```python
from build123d import *

# Parameters (mm, degrees)
PAD002_DEPTH                  = 15.24
SKETCH006_W                   = 33.02
SKETCH006_H                   = 11.684
POCKET003_DEPTH               = 50.8
SKETCH007_R                   = 1.905
POCKET004_DEPTH               = 15.241
SKETCH008_R                   = 1.397
POCKET005_DEPTH               = 12.7
PAD003_DEPTH                  = 0.508
POCKET006_DEPTH               = 13.716
POCKET006_MIRRORED002_2_DEPTH = 13.716
SKETCH011_R                   = 1.016
POCKET007_DEPTH               = 15.749
SKETCH012_R                   = 3.556
SKETCH012_R_2                 = 1.016
SKETCH012_R_3                 = 1.905
PAD004_DEPTH                  = 10.16
SKETCH013_W                   = 2.032
SKETCH013_H                   = 12.7
POCKET008_DEPTH               = 15.749
LINEARPATTERN001_COUNT        = 8
LINEARPATTERN001_PITCH        = 3.628571
POCKET009_DEPTH               = 5.08
POCKET010_DEPTH               = 3.81
SKETCH016_R                   = 3.168854
SKETCH016_W                   = 8.848516
SKETCH016_H                   = 9.89258
POCKET011_DEPTH               = 13.716
SKETCH017_R                   = 3.175
POCKET012_DEPTH               = 5.08
SKETCH018_R                   = 4.445
POCKET013_DEPTH               = 0.9652
SKETCH019_W                   = 5.842
SKETCH019_H                   = 5.08
POCKET014_DEPTH               = 11.43


with BuildPart() as part:
    # Sketch005 → Pad002 (new body)
    with BuildSketch(Plane.XY):
        with BuildLine():
            Line((-37.465, -32.639), (37.465, -32.639))
            ThreePointArc((37.465, -32.639), (42.853154, -30.407154), (45.085, -25.019))
            Line((45.085, -25.019), (45.085, 25.019))
            ThreePointArc((45.085, 25.019), (42.853154, 30.407154), (37.465, 32.639))
            Line((37.465, 32.639), (-37.465, 32.639))
            ThreePointArc((-37.465, 32.639), (-42.853154, 30.407154), (-45.085, 25.019))
            Line((-45.085, 25.019), (-45.085, -25.019))
            ThreePointArc((-45.085, -25.019), (-42.853154, -30.407154), (-37.465, -32.639))
        make_face()
    extrude(amount=PAD002_DEPTH)

    # Sketch006 (on Face3 of Pad002) → Pocket003 (cut)
    with BuildSketch(Plane.YZ.offset(45.085)):
        with Locations((0, 5.842)):
            Rectangle(SKETCH006_W, SKETCH006_H)
    extrude(amount=-POCKET003_DEPTH, mode=Mode.SUBTRACT)

    # Sketch007 (on Face5 of Pocket003) → Pocket004 (cut, through all)
    with BuildSketch(Plane.XY.offset(15.24)):
        with Locations((-24.921036, -19.484434)):
            Circle(SKETCH007_R)
        with Locations((-6.389822, 22.858831)):
            Circle(SKETCH007_R)
        with Locations((17.175787, 27.39946)):
            Circle(SKETCH007_R)
    extrude(amount=-POCKET004_DEPTH, mode=Mode.SUBTRACT)

    # Sketch008 (on Face4 of Pocket004) → Pocket005 (cut)
    with BuildSketch(Plane(origin=(0, 0, 0), x_dir=(1, 0, 0), z_dir=(0, 0, -1))):
        with Locations((37.5, 25)):
            Circle(SKETCH008_R)
        with Locations((37.5, -25)):
            Circle(SKETCH008_R)
        with Locations((-37.5, -25)):
            Circle(SKETCH008_R)
        with Locations((-37.5, 25)):
            Circle(SKETCH008_R)
    extrude(amount=-POCKET005_DEPTH, mode=Mode.SUBTRACT)

    # Sketch009 (on Face4 of Pocket005) → Pad003 (join)
    with BuildSketch(Plane(origin=(0, 0, 0), x_dir=(1, 0, 0), z_dir=(0, 0, -1))):
        with BuildLine():
            Line((-37.5, -31.242), (37.5, -31.242))
            ThreePointArc((37.5, -31.242), (41.913761, -29.413761), (43.742, -25))
            Line((43.742, -25), (43.742, 25))
            ThreePointArc((43.742, 25), (41.913761, 29.413761), (37.5, 31.242))
            Line((37.5, 31.242), (-37.5, 31.242))
            ThreePointArc((-37.5, 31.242), (-41.913761, 29.413761), (-43.742, 25))
            Line((-43.742, 25), (-43.742, -25))
            ThreePointArc((-43.742, -25), (-41.913761, -29.413761), (-37.5, -31.242))
        make_face()
        with BuildLine():
            Line((-37.5, -30.48), (37.5, -30.48))
            ThreePointArc((37.5, -30.48), (41.374945, -28.874945), (42.98, -25))
            Line((42.98, -25), (42.98, 25))
            ThreePointArc((42.98, 25), (41.374945, 28.874945), (37.5, 30.48))
            Line((37.5, 30.48), (-37.5, 30.48))
            ThreePointArc((-37.5, 30.48), (-41.374945, 28.874945), (-42.98, 25))
            Line((-42.98, 25), (-42.98, -25))
            ThreePointArc((-42.98, -25), (-41.374945, -28.874945), (-37.5, -30.48))
        make_face(mode=Mode.SUBTRACT)
    extrude(amount=PAD003_DEPTH)

    # Sketch010 (on Face26 of Pad003) → Pocket006 (cut)
    with BuildSketch(Plane(origin=(0, 0, 0), x_dir=(1, 0, 0), z_dir=(0, 0, -1))):
        with BuildLine():
            ThreePointArc((-37.5, 21.825), (-35.254936, 22.754936), (-34.325, 25))
            Line((-34.325, 25), (0, 25))
            Line((0, 25), (0, 0))
            Line((-37.5, 0), (0, 0))
            Line((-37.5, 21.825), (-37.5, 0))
        make_face()
    pocket006 = extrude(amount=-POCKET006_DEPTH, mode=Mode.SUBTRACT)

    # Sketch010 Mirrored002 2 → Pocket006 Mirrored002 2 (cut)
    with BuildSketch(Plane(origin=(0, 0, 0), x_dir=(-1, 0, 0), z_dir=(0, 0, 1))):
        with BuildLine():
            ThreePointArc((-37.5, 21.825), (-35.254936, 22.754936), (-34.325, 25))
            Line((-34.325, 25), (0, 25))
            Line((0, 25), (0, 0))
            Line((-37.5, 0), (0, 0))
            Line((-37.5, 21.825), (-37.5, 0))
        make_face()
    pocket006_mirrored002_2 = extrude(amount=POCKET006_MIRRORED002_2_DEPTH, mode=Mode.SUBTRACT)

    # Mirrored003: Pocket006, Pocket006 Mirrored002 2 across Sketch010 H_Axis
    add(pocket006.mirror(Plane(origin=(0, 0, 0), x_dir=(0, 0, -1), z_dir=(0, -1, 0))), mode=Mode.SUBTRACT)
    add(pocket006_mirrored002_2.mirror(Plane(origin=(0, 0, 0), x_dir=(0, 0, -1), z_dir=(0, -1, 0))), mode=Mode.SUBTRACT)

    # Sketch011 (on Face5 of MultiTransform001) → Pocket007 (cut, through all)
    with BuildSketch(Plane.XY.offset(15.24)):
        with Locations((-31.977287, 11.541788)):
            Circle(SKETCH011_R)
    extrude(amount=-POCKET007_DEPTH, mode=Mode.SUBTRACT)

    # Sketch012 (on Face31 of Pocket007) → Pad004 (join)
    with BuildSketch(Plane(origin=(0, 0, 13.716), x_dir=(1, 0, 0), z_dir=(0, 0, -1))):
        with Locations((-31.977287, -11.541788)):
            Circle(SKETCH012_R)
        with Locations((-31.977287, -11.541788)):
            Circle(SKETCH012_R_2, mode=Mode.SUBTRACT)
        with Locations((-24.921036, 19.484434)):
            Circle(SKETCH012_R)
        with Locations((-24.921036, 19.484434)):
            Circle(SKETCH012_R_3, mode=Mode.SUBTRACT)
        with Locations((-6.389822, -22.858831)):
            Circle(SKETCH012_R)
        with Locations((-6.389822, -22.858831)):
            Circle(SKETCH012_R_3, mode=Mode.SUBTRACT)
    extrude(amount=PAD004_DEPTH)

    # Sketch013 (on Face5 of Pad004) → Pocket008 (cut, through all)
    with BuildSketch(Plane.XY.offset(15.24)):
        with Locations((0, 16.51)):
            Rectangle(SKETCH013_W, SKETCH013_H)
    pocket008 = extrude(amount=-POCKET008_DEPTH, mode=Mode.SUBTRACT)

    # LinearPattern001: Pocket008 ×8
    with Locations(*[(i * LINEARPATTERN001_PITCH, 0, 0) for i in range(1, LINEARPATTERN001_COUNT)]):
        add(pocket008, mode=Mode.SUBTRACT)

    # Sketch014 (on Face7 of LinearPattern001) → Pocket009 (cut)
    with BuildSketch(Plane.YZ.offset(45.085)):
        Polygon((5.334, 14.732), (5.334, 11.684), (0, 11.684), (0, 0), (0, -2.032), (16.51, -2.032), (16.51, 11.684), (11.176, 11.684), (11.176, 14.732), align=None)
    pocket009 = extrude(amount=-POCKET009_DEPTH, mode=Mode.SUBTRACT)

    # Mirrored004: Pocket009 across Sketch014 V_Axis
    add(pocket009.mirror(Plane(origin=(45.085, 0, 0), x_dir=(1, 0, 0), z_dir=(0, 1, 0))), mode=Mode.SUBTRACT)

    # Sketch015 → Pocket010 (cut, symmetric)
    with BuildSketch(Plane.YZ):
        Polygon((0, 40.386), (-40.386, 0), (-40.386, 3.592102), (-3.592102, 40.386), align=None)
    pocket010 = extrude(amount=POCKET010_DEPTH, both=True, mode=Mode.SUBTRACT)

    # Mirrored005: Pocket010 across XZ
    add(pocket010.mirror(Plane.XZ), mode=Mode.SUBTRACT)

    # Sketch016 (on Face77 of Mirrored005) → Pocket011 (cut)
    with BuildSketch(Plane(origin=(0, 0, 0), x_dir=(1, 0, 0), z_dir=(0, 0, -1))):
        with Locations((8.491343, -25.942871)):
            Circle(SKETCH016_R)
        with Locations((27.06874, -24.191018)):
            Rectangle(SKETCH016_W, SKETCH016_H)
    extrude(amount=-POCKET011_DEPTH, mode=Mode.SUBTRACT)

    # Sketch017 (on Face77 of Pocket011) → Pocket012 (cut)
    with BuildSketch(Plane(origin=(0, 0, 0), x_dir=(1, 0, 0), z_dir=(0, 0, -1))):
        with BuildLine():
            Line((-37.5, -30.48), (37.5, -30.48))
            ThreePointArc((37.5, -30.48), (41.374945, -28.874945), (42.98, -25))
            Line((42.98, -25), (42.98, 25))
            ThreePointArc((42.98, 25), (41.374945, 28.874945), (37.5, 30.48))
            Line((37.5, 30.48), (-37.5, 30.48))
            ThreePointArc((-37.5, 30.48), (-41.374945, 28.874945), (-42.98, 25))
            Line((-42.98, 25), (-42.98, -25))
            ThreePointArc((-42.98, -25), (-41.374945, -28.874945), (-37.5, -30.48))
        make_face()
        with Locations((37.5, -25)):
            Circle(SKETCH017_R, mode=Mode.SUBTRACT)
        with Locations((37.5, 25)):
            Circle(SKETCH017_R, mode=Mode.SUBTRACT)
        with Locations((-37.5, 25)):
            Circle(SKETCH017_R, mode=Mode.SUBTRACT)
        with Locations((-37.5, -25)):
            Circle(SKETCH017_R, mode=Mode.SUBTRACT)
    extrude(amount=-POCKET012_DEPTH, mode=Mode.SUBTRACT)

    # Sketch018 (on Face146 of Pocket012) → Pocket013 (cut)
    with BuildSketch(Plane(origin=(0, 0, 0), x_dir=(1, 0, 0), z_dir=(0, 0, -1))):
        with Locations((-37.5, 25)):
            Circle(SKETCH018_R)
        with Locations((37.5, 25)):
            Circle(SKETCH018_R)
        with Locations((37.5, -25)):
            Circle(SKETCH018_R)
        with Locations((-37.5, -25)):
            Circle(SKETCH018_R)
    extrude(amount=-POCKET013_DEPTH, mode=Mode.SUBTRACT)

    # Sketch019 (on Face14 of Pocket013) → Pocket014 (cut)
    with BuildSketch(Plane.YZ.offset(45.085)):
        with Locations((8.255, 14.224)):
            Rectangle(SKETCH019_W, SKETCH019_H)
    pocket014 = extrude(amount=-POCKET014_DEPTH, mode=Mode.SUBTRACT)

    # Mirrored006: Pocket014 across Sketch019 V_Axis
    add(pocket014.mirror(Plane(origin=(45.085, 0, 0), x_dir=(1, 0, 0), z_dir=(0, 1, 0))), mode=Mode.SUBTRACT)


with BuildPart() as part_1:
    # Body001 placement: moved
    add(part.part.moved(Location((0, 0, 0.635))))


solid = part_1.part
```
Can you work these out from the model? Positions are in its coordinate system, mm. A direction names the side the tool comes from. Give positions to 0.01 mm unless a question says otherwise; leave off trailing zeros. Write each loop counter-clockwise with the first axis right and the second up, starting at its lowest first coordinate (ties: lowest second). Pieces come first, ordered by that corner, then holes. Notation, with made-up numbers: (79, -23) -> (100, -23) arc R18 cw to (100, 1) -> close; hole circle Ø11 at (62.5, 14). An arc over 180 degrees is marked (long way). Write item = value, one per line.
(1) Suppose I cut it at B-B on y = 7. Write out the boundary of the cut face in (x, z) (3 decimals), then the cut area to 3 significant figures.
Worked out:
outline = (-45.085, 0.635) -> (-43.742, 0.635) -> (-43.742, 0.127) -> (-42.98, 0.127) -> (-42.98, 5.715) -> (-37.5, 5.715) -> (-37.5, 14.351) -> (33.655, 14.351) -> (33.655, 15.875) -> (-45.085, 15.875) -> close
area = 197 mm^2
(2) Thinking about a two-plate mould opening in X: for faces 1 (the face through (0.053, -30.716, 13.897)), 2 (the face through (0, 32, 0.635)), 3 (the face through (-42.79, 30.47, 8.15)), which applies, released by +X, released by -X, zero draft, split by the parting line, or undercut?
Worked out:
face_1 = undercut
face_2 = zero draft
face_3 = released by -X
(3) I need wall thicknesses on probe 1 along X at (y, z) = (-25, 5.5) (3 decimals); probe 2 along Y at (x, z) = (-11, 4); probe 3 along Y at (x, z) = (-21, 6). Which ranges of each line are inside material? Lowest first, please. Write a range as from..to.
Worked out:
probe_1 = -45.085..-42.98, -40.675..-38.897, -36.103..-34.325, 34.325..36.103, 38.897..40.675, 42.98..45.085
probe_2 = -32.64..-30.48, 30.48..32.64
probe_3 = -32.64..-25, 25..32.64
(4) I'm going to push flat-ended pins straight in: P1, Ø3.5, axis at y = 27, z = 8, coming from the -X side; P2, Ø1.7, axis at y = -12, z = 2, coming from the +X side; P3, Ø3, axis at x = 32.5, y = 15.5, coming from the -Z side. Where does each tip first touch, or does it pass through?
Worked out:
P1 = -45.08
P2 = -42.98
P3 = 14.35
(5) For faces 4 (the face through (3.81, 30, 13)), 5 (the face through (41.865, 29.462, 0.385)), 6 (the face through (37, 25, 13.335)), which set-ups out of +Z, -Z, +X, -X, +Y, -Y let a thin tool reach every point of the face, with its end or its side?
Worked out:
face_4 = none
face_5 = -Z, +X, +Y
face_6 = -Z
(6) Suppose I cut it at A-A on x = 0. Write out the boundary of the cut face in (y, z) (3 decimals).
Worked out:
outline = (-32.639, 0.635) -> (-31.242, 0.635) -> (-31.242, 0.127) -> (-30.48, 0.127) -> (-30.48, 5.715) -> (-25, 5.715) -> (-25, 14.351) -> (10.16, 14.351) -> (10.16, 15.875) -> (-25.146, 15.875) -> (-32.639, 8.382) -> close; (-32.639, 11.974) -> (-28.738, 15.875) -> (-32.639, 15.875) -> close; (22.86, 14.351) -> (25, 14.351) -> (25, 5.715) -> (30.48, 5.715) -> (30.48, 0.127) -> (31.242, 0.127) -> (31.242, 0.635) -> (32.639, 0.635) -> (32.639, 8.382) -> (25.146, 15.875) -> (22.86, 15.875) -> close; (28.738, 15.875) -> (32.639, 11.974) -> (32.639, 15.875) -> close
(7) Suppose I cut it at C-C on x = -13. Write out the boundary of the cut face in (y, z) (3 decimals).
Worked out:
outline = (-32.639, 0.635) -> (-31.242, 0.635) -> (-31.242, 0.127) -> (-30.48, 0.127) -> (-30.48, 5.715) -> (-25, 5.715) -> (-25, 14.351) -> (25, 14.351) -> (25, 5.715) -> (30.48, 5.715) -> (30.48, 0.127) -> (31.242, 0.127) -> (31.242, 0.635) -> (32.639, 0.635) -> (32.639, 15.875) -> (-32.639, 15.875) -> close
